```python
from build123d import *

# Parameters (mm, degrees)
CUT_EXTRUDE1_DEPTH = 2.5
CHAMFER1_SIZE      = 0.767
CHAMFER2_SIZE      = 0.5
FILLET1_R          = 0.2


with BuildPart() as part:
    # Sketch1 → Revolve1 (revolve)
    with BuildSketch(Plane.XY):
        Polygon((0, 4), (0, 0), (21.1, 0), (21.1, 5.975), (12, 5.975), (12, 3), (8.9, 3), (8.9, 4), align=None)
    revolve(axis=Axis((0, 0, 0), (1, 0, 0)))

    # Sketch2 → Cut-Extrude1 (cut)
    with BuildSketch(Plane(origin=(21.1, 0, 0), x_dir=(0, 0, -1), z_dir=(1, 0, 0))):
        Polygon((0, -2.309401077), (2, -1.154700538), (2, 1.154700538), (0, 2.309401077), (-2, 1.154700538), (-2, -1.154700538), align=None)
    extrude(amount=-CUT_EXTRUDE1_DEPTH, mode=Mode.SUBTRACT)

    # Sketch3 → Cut-Revolve1 (revolve, cut)
    with BuildSketch(Plane(origin=(0, 0, 0), x_dir=(-1, 0, 0), z_dir=(0, 0, -1))):
        Polygon((-18.6, 2), (-18.6, 0), (-17.445299462, 0), align=None)
    revolve(axis=Axis((18.600025, 0, 0), (-1, 0, 0)), mode=Mode.SUBTRACT)

    # Chamfer1
    chamfer1_edges = [part.edges().sort_by_distance(p)[0] for p in [
        (0, -4, 0),
        (8.9, -4, 0),
    ]]
    chamfer(chamfer1_edges, length=CHAMFER1_SIZE)

    # Chamfer2
    chamfer2_edges = [part.edges().sort_by_distance(p)[0] for p in [
        (21.1, -5.975, 0),
    ]]
    chamfer(chamfer2_edges, length=CHAMFER2_SIZE)

    # Fillet1
    fillet1_edges = [part.edges().sort_by_distance(p)[0] for p in [
        (12, -3, 0),
    ]]
    fillet(fillet1_edges, radius=FILLET1_R)


solid = part.part
```
Verification items for the finished model (mm, model axes). A direction names the side the tool comes from. Coordinates: 2 decimals unless noted, no trailing zeros. Write each loop counter-clockwise with the first axis right and the second up, starting at its lowest first coordinate (ties: lowest second). Pieces come first, ordered by that corner, then holes. Notation, with made-up numbers: M 13.5,8.25 L 24.5,8.25 A28 ccw 24.5,30.25 Z; hole C 2,0.25 d6. An arc over 180 degrees is marked long. Answer as a JSON object with one key per item and string values. Group by question number.
(1) Tool access check on faces 5 (the face through (4.398, -0.867, -3.905)), 6 (the face through (21.1, 0.1, -2.4)), 7 (the face through (20, 0, 2)). Record the directions out of +Z, -Z, +X, -X, +Y, -Y that give a thin tool (end or side, any length) a straight path to the whole face; none if there is none.
(2) Material ranges on line 1 (X direction, y = -3.25, z = -3.75); line 2 (X direction, y = -3, z = -1); line 3 (Z direction, x = 17.75, y = 3.5), recorded low to high.
(3) Gauge pin test, flat ends, axial feed: pin 1 (3 mm diameter, centred on x = 7.5, z = 0.5, fed in from +Y); pin 2 (1.5 mm diameter, centred on x = 17, y = -1.5, fed in from +Z). Record the tip position at first contact, or that the pin passes through.
(4) Cross-section at A-A, the plane x = 6. Record the cut outline in (y, z), and give its area (3 significant figures).
(5) Release check for a two-part mould opening along X. For faces 1 (the face through (19.87, -1.74, -0.99)), 2 (the face through (10, -3, 0)), 3 (the face through (12, 3, -3)), 4 (the face through (0, 0, 0)) record: +X half, -X half, draft (parallel to the pull), parting line (faces both ways), or undercut.
Reply:
{
 "1": {"face 5": "-X", "face 6": "+Z, -Z, +X, +Y, -Y", "face 7": "+X"},
 "2": {"line 1": "12 to 21.1", "line 2": "0 to 8.9, 12 to 21.1", "line 3": "-4.84 to 4.84"},
 "3": {"pin 1": "y = 4", "pin 2": "z = 5.93"},
 "4": {"outline": "C 0,0 d8", "area": "50.3 mm²"},
 "5": {"face 1": "draft", "face 2": "undercut", "face 3": "undercut", "face 4": "-X half"}
}
